Read the model definition and answer for the solid it produces. Units are mm, in the model's axes. Face numbers are marked on the shaded views. A direction names the side the tool comes from. Give positions to 0.01 mm unless a question says otherwise; leave off trailing zeros. Order: outer loops, then holes, each group sorted by start corner. A loop starts at its lowest first (then second) coordinate and runs counter-clockwise, first axis right, second up. Notation, with made-up numbers: (46.5, 69) - (76.5, 69) arc R24 cw to (76.5, 91) - close; hole circle Ø9 at (19.5, 59). An arc over 180 degrees is marked (long way). Return JSON: item names as keys, results as strings.
```python
from build123d import *

# Parameters (mm, degrees)
EXTRUDE_1_DEPTH     = 13
SKETCH_4_R          = 1
CUT_EXTRUDE_1_DEPTH = 29.458566373
SKETCH_6_R          = 2.95
EXTRUDE_2_DEPTH     = 4.4


with BuildPart() as part:
    # 草圖1 → 填料-伸長1 (new body)
    with BuildSketch(Plane(origin=(0, 0, 0), x_dir=(0, 0, -1), z_dir=(1, 0, 0))):
        Polygon((11.5, 10.6), (16.5, 10.6), (16.5, 8.6), (11.5, 8.6), (11.5, -8.6), (-11.5, -8.6), (-11.5, 8.6), (-16.5, 8.6), (-16.5, 10.6), (-11.5, 10.6), (-11.5, 15.9), (11.5, 15.9), align=None)
    extrude(amount=EXTRUDE_1_DEPTH)

    # 草圖4 → 除料-伸長1 (cut, through all)
    with BuildSketch(Plane(origin=(0, 10.6, 0), x_dir=(1, 0, 0), z_dir=(0, 1, 0))):
        with Locations(Location((6.5, 14.25, 0), (0, 0, 270))):
            Circle(SKETCH_4_R)
        with Locations(Location((6.5, -14.25, 0), (0, 0, 270))):
            Circle(SKETCH_4_R)
    extrude(amount=-CUT_EXTRUDE_1_DEPTH, mode=Mode.SUBTRACT)

    # 草圖6 → 填料-伸長2 (add)
    with BuildSketch(Plane(origin=(0, 15.9, 0), x_dir=(1, 0, 0), z_dir=(0, 1, 0))):
        with Locations(Location((6.5, -4.87, 0), (0, 0, 90))):
            Circle(SKETCH_6_R)
    extrude(amount=EXTRUDE_2_DEPTH)


solid = part.part
```
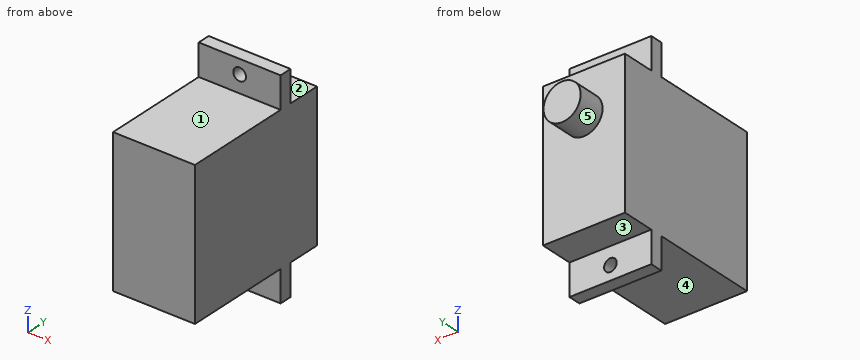
Q1. For the marked faces 1, 2, 3, 4 and 5, determine the directions among +Z, -Z, +X, -X, +Y, -Y from which every point of the face is accessible in a straight line to the end or side of a thin tool.
Values:
{"face 1": "+Z, +X, -X, -Y", "face 2": "+Z, +X, -X, +Y", "face 3": "-Z, +X, -X, +Y", "face 4": "-Z, +X, -X, -Y", "face 5": "+Y"}
Q2. A cutting plane is placed at B-B (z = 14.25). Write down the section's boundary in (x, y).
Values:
{"outline": "(0, 8.6) - (5.5, 8.6) - (5.5, 10.6) - (0, 10.6) - close; (7.5, 8.6) - (13, 8.6) - (13, 10.6) - (7.5, 10.6) - close"}
Q3. Given pin 1 (1.6 mm diameter, centred on x = 5, y = 14, fed in from -Z); pin 2 (1.5 mm diameter, centred on x = 8, z = 14.5, fed in from +Y); pin 3 (4 mm diameter, centred on x = 3.5, y = 13, fed in from +Z), each flat-ended and moving along its own axis, determine where each tip first touches the part or whether it passes through.
Values:
{"pin 1": "stops at z = -11.5", "pin 2": "stops at y = 10.6", "pin 3": "stops at z = 11.5"}
Q4. A cutting plane is placed at D-D (z = 4.87). Write down the section's boundary in (x, y).
Values:
{"outline": "(0, -8.6) - (13, -8.6) - (13, 15.9) - (9.45, 15.9) - (9.45, 20.3) - (3.55, 20.3) - (3.55, 15.9) - (0, 15.9) - close"}
Q5. Consider L1, parallel to X at y = 9.5, z = -14.25; L2, parallel to Y at x = 9.25, z = 3.5; L3, parallel to Y at x = 1.75, z = 13.5. Determine where each line is inside the solid, lowest interval first.
Values:
{"L1": "x = 0 to 5.5, 7.5 to 13", "L2": "y = -8.6 to 15.9", "L3": "y = 8.6 to 10.6"}
Q6. A cutting plane is placed at C-C (x = 2.25). Write down the section's boundary in (y, z), and give its area (4 significant figures).
Values:
{"outline": "(-8.6, -11.5) - (8.6, -11.5) - (8.6, -16.5) - (10.6, -16.5) - (10.6, -11.5) - (15.9, -11.5) - (15.9, 11.5) - (10.6, 11.5) - (10.6, 16.5) - (8.6, 16.5) - (8.6, 11.5) - (-8.6, 11.5) - close", "area": "583.5 mm²"}
Q7. A cutting plane is placed at A-A (x = 6.5). Write down the section's boundary in (y, z).
Values:
{"outline": "(-8.6, -11.5) - (8.6, -11.5) - (8.6, -13.25) - (10.6, -13.25) - (10.6, -11.5) - (15.9, -11.5) - (15.9, 1.92) - (20.3, 1.92) - (20.3, 7.82) - (15.9, 7.82) - (15.9, 11.5) - (10.6, 11.5) - (10.6, 13.25) - (8.6, 13.25) - (8.6, 11.5) - (-8.6, 11.5) - close; (8.6, -16.5) - (10.6, -16.5) - (10.6, -15.25) - (8.6, -15.25) - close; (8.6, 15.25) - (10.6, 15.25) - (10.6, 16.5) - (8.6, 16.5) - close"}
